from build123d import *

# Parameters (mm, degrees)
F0_R     = 12.7
F1_DEPTH = 3.175
F2_R     = 3.75
F3_DEPTH = 12.7
F5_DEPTH = 5.08
F6_DEPTH = 25.4


with BuildPart() as f1:
    # F0 (on Top) → F1 (new body)
    with BuildSketch(Plane.XY):
        Circle(F0_R)
    extrude(amount=F1_DEPTH)

    # F2 (on face) → F3 (join)
    with BuildSketch(Plane.XY.offset(3.175)):
        Circle(F2_R)
    extrude(amount=F3_DEPTH)

    # F4 (on Front) → F5 (cut)
    with BuildSketch(Plane.XZ):
        with BuildLine():
            ThreePointArc((1.6361789283, 12.118075807), (1.7781010103, 12.5127154354), (1.8262548359, 12.929324992))
            ThreePointArc((1.8262548359, 12.929324992), (0.4140579041, 14.7080219245), (-1.6385001539, 13.7358756546))
            ThreePointArc((-1.6385001539, 13.7358756546), (0.4142883311, 14.7027274799), (1.8239336103, 12.9246264696))
            ThreePointArc((1.8239336103, 12.9246264696), (1.7763757069, 12.5105685655), (1.6361789283, 12.118075807))
        make_face()
        with BuildLine():
            ThreePointArc((1.8239336103, 12.9246264696), (0.4142883311, 14.7027274799), (-1.6385001539, 13.7358756546))
            ThreePointArc((-1.6385001539, 13.7358756546), (-0.8089007564, 11.2919837656), (1.6361789283, 12.118075807))
            ThreePointArc((1.6361789283, 12.118075807), (1.7763757069, 12.5105685655), (1.8239336103, 12.9246264696))
        make_face()
        with BuildLine():
            ThreePointArc((1.6361789283, 12.118075807), (-0.8089007564, 11.2919837656), (-1.6385001539, 13.7358756546))
            ThreePointArc((-1.6385001539, 13.7358756546), (-0.811221982, 11.2872852432), (1.6361789283, 12.118075807))
        make_face()
    extrude(amount=F5_DEPTH, mode=Mode.SUBTRACT)

    # F4 (on Front) → F6 (cut)
    with BuildSketch(Plane.XZ):
        with BuildLine():
            ThreePointArc((1.6361789283, 12.118075807), (1.7781010103, 12.5127154354), (1.8262548359, 12.929324992))
            ThreePointArc((1.8262548359, 12.929324992), (0.4140579041, 14.7080219245), (-1.6385001539, 13.7358756546))
            ThreePointArc((-1.6385001539, 13.7358756546), (0.4142883311, 14.7027274799), (1.8239336103, 12.9246264696))
            ThreePointArc((1.8239336103, 12.9246264696), (1.7763757069, 12.5105685655), (1.6361789283, 12.118075807))
        make_face()
        with BuildLine():
            ThreePointArc((1.8239336103, 12.9246264696), (0.4142883311, 14.7027274799), (-1.6385001539, 13.7358756546))
            ThreePointArc((-1.6385001539, 13.7358756546), (-0.8089007564, 11.2919837656), (1.6361789283, 12.118075807))
            ThreePointArc((1.6361789283, 12.118075807), (1.7763757069, 12.5105685655), (1.8239336103, 12.9246264696))
        make_face()
        with BuildLine():
            ThreePointArc((1.6361789283, 12.118075807), (-0.8089007564, 11.2919837656), (-1.6385001539, 13.7358756546))
            ThreePointArc((-1.6385001539, 13.7358756546), (-0.811221982, 11.2872852432), (1.6361789283, 12.118075807))
        make_face()
    extrude(amount=-F6_DEPTH, mode=Mode.SUBTRACT)


solid = f1.part
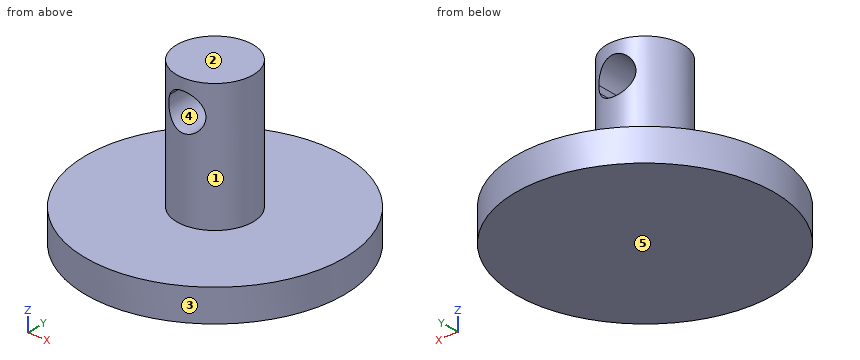
Work out the finished part from the listing and answer in its coordinate system (mm). Face numbers are marked on the shaded views. A direction names the side the tool comes from. Coordinates: 2 decimals unless noted, no trailing zeros. Write each loop counter-clockwise with the first axis right and the second up, starting at its lowest first coordinate (ties: lowest second). Pieces come first, ordered by that corner, then holes. Notation, with made-up numbers: (-0.75, 57.5) - (9.25, 57.5) arc R30 ccw to (9.25, 85.5) - close; hole circle Ø2 at (84, -9.75). An arc over 180 degrees is marked (long way). One line per question, with ' | ' between items.
1) The mould has two halves that part along X. Classify the marked faces 3, 4 and 5: +X half, -X half, draft (parallel to the pull), parting line (faces both ways), or undercut.
Checks:
face 3: parting line | face 4: undercut | face 5: draft
2) Consider probe 1 along Z at (x, y) = (1.75, -6.5) (3 decimals); probe 2 along Z at (x, y) = (0.25, -0.25) (3 decimals); probe 3 along X at (y, z) = (-3, 14.5). Determine where each line is inside the solid, lowest interval first. Write a range as [from, to].
Checks:
probe 1: [0, 3.175] | probe 2: [0, 11.116], [14.738, 15.875] | probe 3: [-2.25, -0.93], [0.93, 2.25]
3) For the marked faces 1 and 2, determine the directions among +Z, -Z, +X, -X, +Y, -Y from which every point of the face is accessible in a straight line to the end or side of a thin tool.
Checks:
face 1: +Z | face 2: +Z, +X, -X, +Y, -Y
4) Find section D-D, the plane z = 3.5. Determine the outline of the cut face in (x, y), and give its area (3 significant figures).
Checks:
outline: circle Ø7.5 at (0, 0) | area: 44.2 mm2
5) Find section A-A, the plane x = 0. Determine the outline of the cut face in (y, z) (3 decimals), and give its area (3 significant figures).
Checks:
outline: (-12.7, 0) - (12.7, 0) - (12.7, 3.175) - (3.75, 3.175) - (3.75, 11.098) - (-3.75, 11.098) - (-3.75, 3.175) - (-12.7, 3.175) - close; (-3.75, 14.756) - (3.75, 14.756) - (3.75, 15.875) - (-3.75, 15.875) - close | area: 148 mm2
6) Find section C-C, the plane z = 11.75. Determine the outline of the cut face in (x, y).
Checks:
outline: (-1.4, -3.48) - (-1.4, 3.48) arc R3.75 ccw to start; (1.4, -3.48) arc R3.75 ccw to (1.4, 3.48) - close
7) Flat-ended cylindrical pins translate along their axes: P1, Ø3, axis at x = -7.5, y = 6.5, coming from the +Z side (3 decimals); P2, Ø1, axis at y = -1, z = 13.5, coming from the +X side. Find the tip coordinate at first contact, or state that the pin passes through.
Checks:
P1: z = 3.175 | P2: x = 3.72
